Geometry check sheet. Reference: the model listing, model coordinates, mm. Face numbers are marked on the shaded views. A direction names the side the tool comes from. Round coordinates to 2 decimals unless told otherwise and drop trailing zeros. Order: outer loops, then holes, each group sorted by start corner. A loop starts at its lowest first (then second) coordinate and runs counter-clockwise, first axis right, second up.
(1) Thickness scan on L1, parallel to Y at x = 210, z = 0 (1 decimal); L2, parallel to Y at x = 128.5, z = 0 (3 decimals); L3, parallel to Z at x = 42.5, y = -1. Record the ranges inside material, lowest first.
(2) Cross-section at B-B on y = 0. Enter the section's corners in (x, z) (3 decimals).
(3) Draft check along Z on the marked faces 1, 2 and 3. Enter one of: pulls with the +Z half, pulls with the -Z half, needs draft (parallel to the pull), parting line crosses it, or undercut.
(4) Set-up check for the marked faces 4 and 5: record each of +Z, -Z, +X, -X, +Y, -Y from which the full face is reachable in a straight line by a thin tool's end or side.
(5) Cross-section at D-D on x = 161. Enter the section's corners in (y, z) (3 decimals).
(6) Cross-section at C-C on x = 109.22. Enter the section's corners in (y, z) (3 decimals).
(7) Cross-section at A-A on z = 4. Count the separate pieces of the cut face and the enclosed holes in it, and give its area (3 significant figures).
(8) Gauge pin test, flat ends, axial feed: P1, Ø2, axis at x = 39, y = 24, coming from the +Z side; P2, Ø13, axis at y = 0, z = 0, coming from the -X side; P3, Ø8, axis at x = 180.5, z = -9, coming from the -Y side; P4, Ø10, axis at x = 57, z = -8, coming from the -Y side. Record the tip position at first contact, or that the pin passes through.
from build123d import *

# Parameters (mm, degrees)
SKETCH1_R                 = 31.75
SKETCH1_R_2               = 10.795
BOSS_EXTRUDE1_DEPTH       = 106.68
SKETCH2_R                 = 12.7
CUT_EXTRUDE1_DEPTH        = 15.875
CUT_EXTRUDE2_START        = -81.28
SKETCH3_OUTSIDE_W         = 111.798
SKETCH3_OUTSIDE_H         = 111.798
SKETCH3_OUTSIDE_R         = 25.4
CUT_EXTRUDE2_DEPTH        = 50.8
CUT_EXTRUDE3_DEPTH        = 25.4
CUT_EXTRUDE3_DEPTH_BACK   = 25.4
SKETCH5_R                 = 3.96875
M4X0_7_TAPPED_HOLE1_D     = 3.3
M4X0_7_TAPPED_HOLE1_DEPTH = 9.906
M4X0_7_TAPPED_HOLE1_TIP   = 0.991420021
SKETCH11_OUTSIDE_W        = 111.798
SKETCH11_OUTSIDE_H        = 111.798
SKETCH11_OUTSIDE_R        = 28.575
CUT_EXTRUDE4_DEPTH        = 6.35


with BuildPart() as part:
    # Sketch1 → Boss-Extrude1 (new body)
    with BuildSketch(Plane(origin=(0, 0, 0), x_dir=(0, 0, -1), z_dir=(1, 0, 0))):
        Circle(SKETCH1_R)
        Circle(SKETCH1_R_2, mode=Mode.SUBTRACT)
    boss_extrude1 = extrude(amount=BOSS_EXTRUDE1_DEPTH)

    # Sketch2 → Cut-Extrude1 (cut)
    with BuildSketch(Plane.ZY):
        Circle(SKETCH2_R)
    cut_extrude1 = extrude(amount=-CUT_EXTRUDE1_DEPTH, mode=Mode.SUBTRACT)

    # Mirror1: Boss-Extrude1, Cut-Extrude1 across plane
    add(boss_extrude1.mirror(Plane(origin=(106.68, 0, 0), x_dir=(0, 0, 1), z_dir=(1, 0, 0))))
    add(cut_extrude1.mirror(Plane(origin=(106.68, 0, 0), x_dir=(0, 0, 1), z_dir=(1, 0, 0))), mode=Mode.SUBTRACT)

    # Sketch3 outside → Cut-Extrude2 (cut)
    with BuildSketch(Plane.ZY.offset(CUT_EXTRUDE2_START)):
        Rectangle(SKETCH3_OUTSIDE_W, SKETCH3_OUTSIDE_H)
        Circle(SKETCH3_OUTSIDE_R, mode=Mode.SUBTRACT)
    extrude(amount=-CUT_EXTRUDE2_DEPTH, mode=Mode.SUBTRACT)

    # Sketch5 → Cut-Extrude3 (cut, two sides: drawn at the far end of the back side and taken through both)
    with BuildSketch(Plane.XY.offset(-CUT_EXTRUDE3_DEPTH_BACK)):
        with Locations(Location((109.22, -17.4625, 0), (0, 0, 180))):
            Circle(SKETCH5_R)
    extrude(amount=CUT_EXTRUDE3_DEPTH + CUT_EXTRUDE3_DEPTH_BACK, mode=Mode.SUBTRACT)

    # M4x0.7 Tapped Hole1
    with Locations(Plane(origin=(213.36, 0, 0), x_dir=(0, 0, -1), z_dir=(1, 0, 0))):
        with Locations((20.622229928, -11.90625), (0, -23.8125), (20.622229928, 11.90625), (0, 23.8125), (-20.622229928, 11.90625), (-20.622229928, -11.90625)):
            Hole(M4X0_7_TAPPED_HOLE1_D / 2, depth=M4X0_7_TAPPED_HOLE1_DEPTH)
            with Locations((0, 0, -(M4X0_7_TAPPED_HOLE1_DEPTH + M4X0_7_TAPPED_HOLE1_TIP / 2))):  # 118° drill point
                Cone(0, M4X0_7_TAPPED_HOLE1_D / 2, M4X0_7_TAPPED_HOLE1_TIP, mode=Mode.SUBTRACT)

    # Sketch11 outside → Cut-Extrude4 (cut)
    with BuildSketch(Plane(origin=(213.36, 0, 0), x_dir=(0, 0, -1), z_dir=(1, 0, 0))):
        Rectangle(SKETCH11_OUTSIDE_W, SKETCH11_OUTSIDE_H)
        Circle(SKETCH11_OUTSIDE_R, mode=Mode.SUBTRACT)
    extrude(amount=-CUT_EXTRUDE4_DEPTH, mode=Mode.SUBTRACT)


solid = part.part
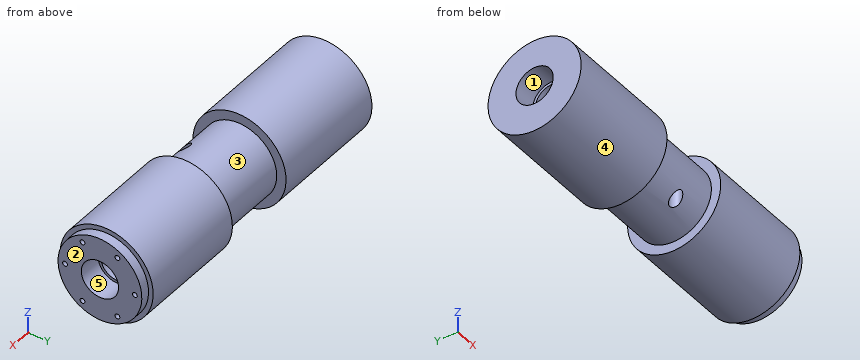
Found:
1. L1: y = -28.6 to -25.5, -22.2 to -12.7, 12.7 to 22.2, 25.5 to 28.6
1. L2: y = -25.4 to -10.795, 10.795 to 25.4
1. L3: z = -31.73 to -10.75, 10.75 to 31.73
2. outline: (0, -31.75) - (81.28, -31.75) - (81.28, -25.4) - (132.08, -25.4) - (132.08, -31.75) - (207.01, -31.75) - (207.01, -28.575) - (213.36, -28.575) - (213.36, -12.7) - (197.485, -12.7) - (197.485, -10.795) - (15.875, -10.795) - (15.875, -12.7) - (0, -12.7) - close; (0, 12.7) - (15.875, 12.7) - (15.875, 10.795) - (197.485, 10.795) - (197.485, 12.7) - (213.36, 12.7) - (213.36, 28.575) - (207.01, 28.575) - (207.01, 31.75) - (132.08, 31.75) - (132.08, 25.4) - (81.28, 25.4) - (81.28, 31.75) - (0, 31.75) - close
3. face 1: undercut
3. face 2: needs draft
3. face 3: parting line crosses it
4. face 4: +X, -X
4. face 5: +X
5. outline: circle Ø63.5 at (0, 0); hole circle Ø21.59 at (0, 0)
6. outline: (-21.431, -13.633) - (-21.431, 13.633) arc R25.4 ccw to start; (-13.494, -21.519) arc R25.4 ccw (long way) to (-13.494, 21.519) - close; hole circle Ø21.59 at (0, 0)
7. separate pieces: 2
7. enclosed holes: 1
7. area: 8,290 mm2
8. P1: stops at z = 21.89
8. P2: passes through
8. P3: stops at y = -31.35
8. P4: stops at y = -31.61
